Geometry check sheet. Reference: the model listing, model coordinates, mm. A direction names the side the tool comes from. Give positions to 0.01 mm unless a question says otherwise; leave off trailing zeros. Loops run counter-clockwise (first coordinate to the right, second up) from the corner with the lowest first, then second, coordinate; pieces in that order, holes last. Notation, with made-up numbers: (60, 64.5) -> (91, 64.5) arc R17 cw to (91, 97.5) -> close; hole circle Ø11 at (79, -31.5). An arc over 180 degrees is marked (long way). Answer in a Markdown table with one row per item. Add a question column.
```python
from build123d import *

# Parameters (mm, degrees)
BOSS_EXTRUDE1_DEPTH = 17.5
SKETCH6_W           = 24.942027916
SKETCH6_H           = 10
SKETCH6_W_2         = 47.258134024
SKETCH6_H_2         = 13
SKETCH6_H_3         = 12
SKETCH6_W_3         = 26
CUT_EXTRUDE1_DEPTH  = 228.033901494
SKETCH7_R           = 25
CUT_EXTRUDE2_DEPTH  = 228.033901494
SKETCH8_R           = 4
CUT_EXTRUDE3_DEPTH  = 30
SKETCH10_R          = 4
CUT_EXTRUDE4_DEPTH  = 30
SKETCH11_W          = 7.160304618
SKETCH11_H          = 39.552070702
SKETCH11_H_2        = 22.637315958
BOSS_EXTRUDE2_DEPTH = 50
SKETCH13_R          = 4
CUT_EXTRUDE5_DEPTH  = 50
CUT_EXTRUDE6_DEPTH  = 50
CUT_EXTRUDE7_DEPTH  = 50
BOSS_EXTRUDE3_DEPTH = 70
SKETCH19_R          = 4
CUT_EXTRUDE8_DEPTH  = 70
FILLET4_R           = 5
CUT_EXTRUDE11_DEPTH = 250.744819662
FILLET5_R           = 3
FILLET6_R           = 3
CUT_EXTRUDE12_DEPTH = 250.744819662
FILLET9_R           = 3
CUT_EXTRUDE13_DEPTH = 247.600171616
FILLET10_R          = 3
CUT_EXTRUDE14_DEPTH = 50
FILLET11_R          = 4
CUT_EXTRUDE16_DEPTH = 100


with BuildPart() as part:
    # Sketch1 → Boss-Extrude1 (new, symmetric)
    with BuildSketch(Plane.XY):
        Polygon((30, -10), (-30, -10), (-30, 140), (-43.810871114, 190), (-43.810871114, 220), (-13.810871114, 220), (-13.810871114, 190), (30, 140), align=None)
    extrude(amount=BOSS_EXTRUDE1_DEPTH, both=True)

    # Sketch6 → Cut-Extrude1 (cut, through all)
    with BuildSketch(Plane(origin=(0, 0, -17.5), x_dir=(-1, 0, 0), z_dir=(0, 0, -1))):
        with Locations((28.506361164, 188.88472005)):
            Rectangle(SKETCH6_W, SKETCH6_H)
        Rectangle(SKETCH6_W_2, SKETCH6_H_2)
        with Locations((0, 17.5)):
            Rectangle(SKETCH6_W_2, SKETCH6_H_3)
        with Locations((28.85405418, 205.307263481)):
            Rectangle(SKETCH6_W_3, SKETCH6_H_2)
    extrude(amount=-CUT_EXTRUDE1_DEPTH, mode=Mode.SUBTRACT)

    # Sketch7 → Cut-Extrude2 (cut, through all)
    with BuildSketch(Plane(origin=(0, 0, -17.5), x_dir=(-1, 0, 0), z_dir=(0, 0, -1))):
        with Locations((0, 105)):
            Circle(SKETCH7_R)
    extrude(amount=-CUT_EXTRUDE2_DEPTH, mode=Mode.SUBTRACT)

    # Sketch8 → Cut-Extrude3 (cut)
    with BuildSketch(Plane(origin=(0, 220, 0), x_dir=(1, 0, 0), z_dir=(0, 1, 0))):
        with Locations(Location((-28.860081831, 7.158757746, 0), (0, 0, 270))):
            Circle(SKETCH8_R)
    extrude(amount=-CUT_EXTRUDE3_DEPTH, mode=Mode.SUBTRACT)

    # Sketch10 → Cut-Extrude4 (cut)
    with BuildSketch(Plane.XZ.offset(10)):
        Circle(SKETCH10_R)
    extrude(amount=-CUT_EXTRUDE4_DEPTH, mode=Mode.SUBTRACT)

    # Sketch11 → Boss-Extrude2 (add)
    with BuildSketch(Plane(origin=(30, 0, 0), x_dir=(0, 0, -1), z_dir=(1, 0, 0))):
        with Locations((-0.000773436, 90.343921661)):
            Rectangle(SKETCH11_W, SKETCH11_H)
        with Locations((-0.000773436, 32.969473472)):
            Rectangle(SKETCH11_W, SKETCH11_H_2)
    extrude(amount=BOSS_EXTRUDE2_DEPTH)

    # Sketch13 → Cut-Extrude5 (cut)
    with BuildSketch(Plane.XY.offset(3.580925745)):
        with Locations((69.802457577, 90.343921661)):
            Circle(SKETCH13_R)
        with Locations((42.591748381, 32.969473472)):
            Circle(SKETCH13_R)
    extrude(amount=-CUT_EXTRUDE5_DEPTH, mode=Mode.SUBTRACT)

    # Sketch14 → Cut-Extrude6 (cut)
    with BuildSketch(Plane.XY.offset(3.580925745)):
        with BuildLine():
            Line((30, 110.119957012), (71.857382865, 97.843921661))
            ThreePointArc((71.857382865, 97.843921661), (77.47366635, 90.343921661), (71.857382865, 82.843921661))
            Line((71.857382865, 82.843921661), (30, 70.56788631))
            Line((30, 70.56788631), (80, 70.56788631))
            Line((80, 70.56788631), (80, 110.119957012))
            Line((80, 110.119957012), (30, 110.119957012))
        make_face()
    extrude(amount=-CUT_EXTRUDE6_DEPTH, mode=Mode.SUBTRACT)

    # Sketch15 → Cut-Extrude7 (cut)
    with BuildSketch(Plane.XY.offset(3.580925745)):
        with BuildLine():
            Line((30, 44.288131451), (80, 44.288131451))
            Line((80, 44.288131451), (80, 21.650815493))
            Line((80, 21.650815493), (30, 21.650815493))
            Line((30, 21.650815493), (45.536546747, 27.022566957))
            ThreePointArc((45.536546747, 27.022566957), (49.751512, 32.928989945), (45.556761025, 38.849786248))
            Line((45.556761025, 38.849786248), (30, 44.288131451))
        make_face()
    extrude(amount=-CUT_EXTRUDE7_DEPTH, mode=Mode.SUBTRACT)

    # Sketch18 → Boss-Extrude3 (add)
    with BuildSketch(Plane.ZY.offset(30)):
        Polygon((11.672732765, 47), (-11.672732765, 47), (-45.527572918, 47), (-45.527572918, 42), (-11.672732765, 42), (11.672732765, 42), align=None)
        Polygon((-11.672732765, 26), (-45.212973929, 26), (-45.212973929, 21), (-11.672732765, 21), (11.672732765, 21), (11.672732765, 26), align=None)
    extrude(amount=BOSS_EXTRUDE3_DEPTH)

    # Sketch19 → Cut-Extrude8 (cut)
    with BuildSketch(Plane(origin=(0, 47, 0), x_dir=(1, 0, 0), z_dir=(0, 1, 0))):
        with Locations(Location((-85, 33, 0), (0, 0, 270))):
            Circle(SKETCH19_R)
    extrude(amount=-CUT_EXTRUDE8_DEPTH, mode=Mode.SUBTRACT)

    # Fillet4
    fillet4_edges = [part.edges().sort_by_distance(p)[0] for p in [
        (-40.977375122, 183.88472005, 0),
        (-16.035347206, 183.88472005, 0),
        (-16.035347206, 193.88472005, 0),
        (-40.977375122, 193.88472005, 0),
    ]]
    fillet(fillet4_edges, radius=FILLET4_R - 0.0001)  # a hair under: the kernel refuses the full size

    # Sketch24 → Cut-Extrude11 (cut, through all)
    with BuildSketch(Plane.XY.offset(17.5)):
        Polygon((-23.080104547, 29.96241896), (-23.080104547, 72.243295408), (19.739020818, 29.96241896), align=None)
        Polygon((-16.517242483, 72.243295408), (23.954637672, 72.243295408), (23.954637672, 32.280158612), align=None)
    extrude(amount=-CUT_EXTRUDE11_DEPTH, mode=Mode.SUBTRACT)

    # Fillet5
    fillet5_edges = [part.edges().sort_by_distance(p)[0] for p in [
        (-16.517242483, 72.243295408, 0),
        (23.954637672, 72.243295408, 0),
    ]]
    fillet(fillet5_edges, radius=FILLET5_R)

    # Fillet6
    fillet6_edges = [part.edges().sort_by_distance(p)[0] for p in [
        (23.954637672, 32.280158612, 0),
        (19.739020818, 29.96241896, 0),
        (-23.080104547, 29.96241896, 0),
        (-23.080104547, 72.243295408, 0),
    ]]
    fillet(fillet6_edges, radius=FILLET6_R)

    # Sketch25 → Cut-Extrude12 (cut, through all)
    with BuildSketch(Plane.XY.offset(17.5)):
        with BuildLine():
            Line((19.626327343, 134.005049283), (-12.289470121, 176.922125419))
            Line((-12.289470121, 176.922125419), (-30.503104083, 176.922125419))
            Line((-30.503104083, 176.922125419), (-20.751992176, 132.120430764))
            ThreePointArc((-20.751992176, 132.120430764), (-0.889923513, 140.07073059), (19.626327343, 134.005049283))
        make_face()
    extrude(amount=-CUT_EXTRUDE12_DEPTH, mode=Mode.SUBTRACT)

    # Fillet9
    fillet9_edges = [part.edges().sort_by_distance(p)[0] for p in [
        (19.626327343, 134.005049283, 0),
        (-20.751992176, 132.120430764, 0),
        (-30.503104083, 176.922125419, 0),
        (-12.289470121, 176.922125419, 0),
    ]]
    fillet(fillet9_edges, radius=FILLET9_R)

    # Sketch26 → Cut-Extrude13 (cut, through all)
    with BuildSketch(Plane.XY.offset(3.580925745)):
        with BuildLine():
            Line((30, 101.953158871), (56.185596991, 94.877842692))
            ThreePointArc((56.185596991, 94.877842692), (59.655725238, 90.345648843), (56.185596991, 85.813454995))
            Line((56.185596991, 85.813454995), (30, 77.952755802))
            Line((30, 77.952755802), (30, 101.953158871))
        make_face()
    extrude(amount=-CUT_EXTRUDE13_DEPTH, mode=Mode.SUBTRACT)

    # Fillet10
    fillet10_edges = [part.edges().sort_by_distance(p)[0] for p in [
        (23.629067012, -6.5, 0),
        (23.629067012, 6.5, 0),
        (-23.629067012, 6.5, 0),
        (-23.629067012, -6.5, 0),
        (-15.85405418, 198.807263481, 0),
        (-15.85405418, 211.807263481, 0),
        (-41.85405418, 211.807263481, 0),
        (-41.85405418, 198.807263481, 0),
        (23.629067012, 11.5, 0),
        (23.629067012, 23.5, 0),
        (-23.629067012, 23.5, 0),
        (-23.629067012, 11.5, 0),
    ]]
    fillet(fillet10_edges, radius=FILLET10_R)

    # Sketch29 → Cut-Extrude14 (cut)
    with BuildSketch(Plane.XZ.offset(-21)):
        with BuildLine():
            Line((-30, 4.855454999), (-90.46980655, -27.217712952))
            ThreePointArc((-90.46980655, -27.217712952), (-93.474418669, -37.006897491), (-83.685693812, -40.01300687))
            Line((-83.685693812, -40.01300687), (-30, -11.55916998))
            Line((-30, -11.55916998), (-30, -45.527572918))
            Line((-30, -45.527572918), (-100, -45.527572918))
            Line((-100, -45.527572918), (-100, 11.672732765))
            Line((-100, 11.672732765), (-30, 11.672732765))
            Line((-30, 11.672732765), (-30, 4.855454999))
        make_face()
    extrude(amount=-CUT_EXTRUDE14_DEPTH, mode=Mode.SUBTRACT)

    # Fillet11
    fillet11_edges = [part.edges().sort_by_distance(p)[0] for p in [
        (-30, 140, 0),
        (-43.810871114, 190, 0),
        (-13.810871114, 190, 0),
        (30, 140, 0),
    ]]
    fillet(fillet11_edges, radius=FILLET11_R)

    # Sketch31 → Cut-Extrude16 (cut)
    with BuildSketch(Plane(origin=(30, 0, 0), x_dir=(0, 0, -1), z_dir=(1, 0, 0))):
        Polygon((-17.5, 141.131578769), (-2.764763692, 188.868421231), (-2.764763692, 220), (-17.5, 220), align=None)
    extrude(amount=-CUT_EXTRUDE16_DEPTH, mode=Mode.SUBTRACT)


solid = part.part
```
1. Release check for a two-part mould opening along X. For faces 5 (the face through (-20, 176.922, -5)), 6 (the face through (-62, 21, -20)), 7 (the face through (-59.812, 23.465, -10.957)) record: released by +X, released by -X, zero draft, split by the parting line, or undercut.
2. Material ranges on L1, parallel to X at y = 91.5, z = -5.5; L2, parallel to Y at x = 16.5, z = -7.5; L3, parallel to Z at x = 0, y = 8.8, recorded low to high. Write a range as from..to.
3. Sectioned sample at B-B (x = 35). Enter the section's corners in (y, z), plus the area to 3 significant figures.
4. Gauge pin test, flat ends, axial feed: pin 1 Ø10 at (x, z) = (-49, -29.5) entering from -Y; pin 2 Ø2 at (y, z) = (1, -0.5) entering from +X; pin 3 Ø20 at (x, y) = (47, 92) entering from +Z; pin 4 Ø1.5 at (y, z) = (129.5, 5) entering from -X. Record the tip position at first contact, or that the pin passes through.
5. Sectioned sample at A-A (y = 17.5). Enter the section's corners in (x, z), plus the area to 3 significant figures.
6. Sectioned sample at C-C (z = -33). Enter the section's corners in (x, y), plus the area to 3 significant figures.
7. Sectioned sample at D-D (x = -62). Enter the section's corners in (y, z), plus the area to 3 significant figures.
8. Access from +Z, -Z, +X, -X, +Y, -Y to the whole of each face (thin tool, end or side, straight path). Record for faces 1 (the face through (-43.811, 205, -7)), 2 (the face through (-57.219, 23.465, -25.985)), 3 (the face through (-0.867, 8.965, -3.905)), 4 (the face through (22.066, 36.672, -0.245)).
Response:
| question | item | result |
|---|---|---|
| 1 | face 5 | undercut |
| 1 | face 6 | zero draft |
| 1 | face 7 | released by -X |
| 2 | L1 | x = -30..-21.04, 21.04..30 |
| 2 | L2 | y = -10..-6.5, 6.5..11.5, 23.5..39.64, 72.24..86.22, 123.78..155.41 |
| 2 | L3 | z = -17.5..-4, 4..17.5 |
| 3 | outline | (23.38, -3.58) -> (42.54, -3.58) -> (42.54, 3.58) -> (23.38, 3.58) -> close; (72.03, -3.58) -> (79.45, -3.58) -> (79.45, 3.58) -> (72.03, 3.58) -> close; (100.6, -3.58) -> (108.65, -3.58) -> (108.65, 3.58) -> (100.6, 3.58) -> close |
| 3 | area | 248 mm2 |
| 4 | pin 1 | passes through |
| 4 | pin 2 | stops at x = 30 |
| 4 | pin 3 | stops at z = 3.58 |
| 4 | pin 4 | stops at x = -30 |
| 5 | outline | (-30, -17.5) -> (-23.63, -17.5) -> (-23.63, 17.5) -> (-30, 17.5) -> close; (23.63, -17.5) -> (30, -17.5) -> (30, 17.5) -> (23.63, 17.5) -> close |
| 5 | area | 446 mm2 |
| 6 | outline | (-94.29, 21) -> (-89, 21) -> (-89, 26) -> (-94.29, 26) -> close; (-94.29, 42) -> (-89, 42) -> (-89, 47) -> (-94.29, 47) -> close; (-81, 21) -> (-70.45, 21) -> (-70.45, 26) -> (-81, 26) -> close; (-81, 42) -> (-70.45, 42) -> (-70.45, 47) -> (-81, 47) -> close |
| 6 | area | 158 mm2 |
| 7 | outline | (21, -28.52) -> (26, -28.52) -> (26, -12.12) -> (21, -12.12) -> close; (42, -28.52) -> (47, -28.52) -> (47, -12.12) -> (42, -12.12) -> close |
| 7 | area | 164 mm2 |
| 8 | face 1 | +Z, -Z, -X, +Y |
| 8 | face 2 | -Z, -Y |
| 8 | face 3 | -Y |
| 8 | face 4 | +Z, -Z |
